Geometry: final body of the model. Coordinates: model frame, mm. Face numbers are marked on the shaded views. A direction names the side the tool comes from. Coordinates: 2 decimals unless noted, no trailing zeros. Write each loop counter-clockwise with the first axis right and the second up, starting at its lowest first coordinate (ties: lowest second). Pieces come first, ordered by that corner, then holes. Notation, with made-up numbers: (-38, -12) -> (-25, -12) arc R18 cw to (-25, -7) -> close; hole circle Ø11 at (21, 68). An arc over 180 degrees is marked (long way). One line per item, written item: value.
```python
from build123d import *

# Parameters (mm, degrees)
F1_DEPTH = 10
F4_SIZE  = 5


with BuildPart() as f1:
    # F0 (on Top) → F1 (new body)
    with BuildSketch(Plane.XY):
        Polygon((-25, 14.4337567297), (-25, -14.4337567297), (0, -28.8675134595), (25, -14.4337567297), (25, 14.4337567297), (0, 28.8675134595), align=None)
    extrude(amount=F1_DEPTH)

    # F2 (on Front) → F3 (revolve)
    with BuildSketch(Plane.XZ):
        with BuildLine():
            Line((0, 10), (0, 30))
            ThreePointArc((0, 30), (-3.5846514013, 30.6645688728), (-6.6928532543, 32.5699451337))
            ThreePointArc((-6.6928532543, 32.5699451337), (-5.9483456169, 20.9335846587), (-10, 10))
            Line((-10, 10), (0, 10))
        make_face()
        with BuildLine():
            Line((0, 30), (0, 50))
            ThreePointArc((0, 50), (-7.0710678119, 47.0710678119), (-10, 40))
            ThreePointArc((-10, 40), (-8.0756928824, 36.4054772252), (-6.6928532543, 32.5699451337))
            ThreePointArc((-6.6928532543, 32.5699451337), (-3.5846514013, 30.6645688728), (0, 30))
        make_face()
        with BuildLine():
            ThreePointArc((-6.6928532543, 32.5699451337), (-8.0756928824, 36.4054772252), (-10, 40))
            ThreePointArc((-10, 40), (-9.1358779694, 35.9335846587), (-6.6928532543, 32.5699451337))
        make_face()
    revolve(axis=Axis((0, 0, 30), (0, 0, 1)))

    # F4
    f4_edges = [f1.edges().sort_by_distance(p)[0] for p in [
        (-25, 0, 10),
        (-12.5, -21.650635, 10),
        (-12.5, 21.650635, 10),
        (12.5, 21.650635, 10),
        (25, 0, 10),
        (12.5, -21.650635, 10),
    ]]
    chamfer(f4_edges, length=F4_SIZE)


solid = f1.part
```
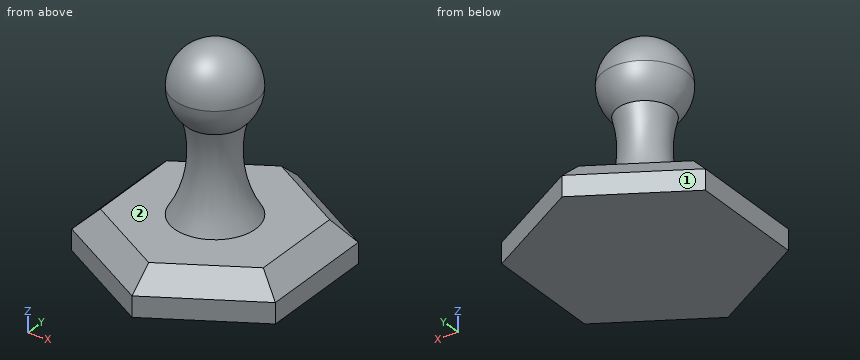
(1) Reachability of the marked faces 1 and 2 from +Z, -Z, +X, -X, +Y, -Y: full face, straight path, thin tool, end or side. Return the list, or none.
Responses:
face 1: +Z, -Z, -X, +Y
face 2: +Z
(2) Section C-C (z = 30.5). Return the cut outline in (x, y).
Responses:
outline: circle Ø12.39 at (0, 0)
(3) Line query: line 1 (Z direction, x = 4, y = 8); line 2 (Z direction, x = 2, y = 16); line 3 (Y direction, x = -19, z = 8). Output: solid intervals per line, ascending. Write a range as [from, to].
Responses:
line 1: z = [0, 11.82], [35.53, 44.47]
line 2: z = [0, 10]
line 3: y = [-14.43, 14.43]
(4) First-contact query: pin 1 (2 mm diameter, centred on y = 11, z = 13, fed in from -X); pin 2 (10 mm diameter, centred on x = 3, z = 34.5, fed in from +Y); pin 3 (6 mm diameter, centred on x = -9.5, z = 42, fed in from +Y); pin 4 (6 mm diameter, centred on x = -17, z = 7, fed in from +Y). Flat tips, straight axial feed; report the tip coordinate or a pass-through.
Responses:
pin 1: passes through
pin 2: stops at y = 9.92
pin 3: stops at y = 7.42
pin 4: stops at y = 20.34
(5) Section A-A (x = 11). Return the cut outline in (y, z).
Responses:
outline: (-22.52, 0) -> (22.52, 0) -> (22.52, 5) -> (16.74, 10) -> (-16.74, 10) -> (-22.52, 5) -> close
(6) Section B-B (y = 21.5). Return the cut outline in (x, z), then the cut area to 3 significant figures.
Responses:
outline: (-12.76, 0) -> (12.76, 0) -> (12.76, 5) -> (2.76, 10) -> (-2.76, 10) -> (-12.76, 5) -> close
area: 205 mm2
